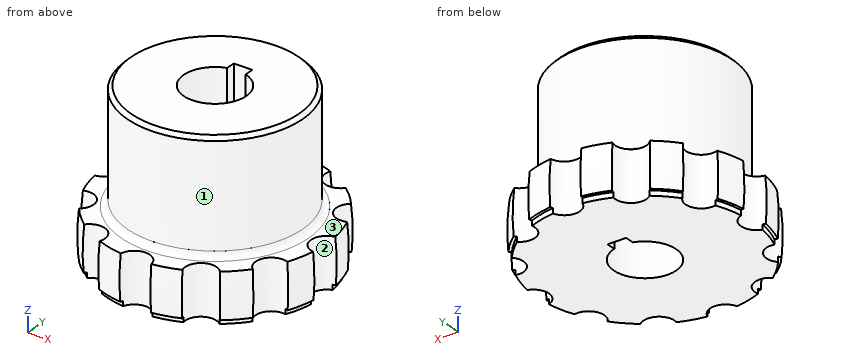
from build123d import *

# Parameters (mm, degrees)
SKETCH_1_R          = 130
EXTRUDE_1_DEPTH     = 40
SKETCH_2_R          = 70
EXTRUDE_2_DEPTH     = 130
SKETCH_4_R          = 12.5
CUT_EXTRUDE_1_DEPTH = 70
FILLET_1_R          = 5
CHAMFER_1_SIZE      = 3
SCALE_1_SCALE       = 0.2
CUT_EXTRUDE_3_DEPTH = 37.215474988


with BuildPart() as part:
    # 草图1 → 凸台-拉伸1 (new body)
    with BuildSketch(Plane.XY):
        Circle(SKETCH_1_R)
    extrude(amount=EXTRUDE_1_DEPTH)

    # 草图2 → 凸台-拉伸2 (add)
    with BuildSketch(Plane.XY):
        Circle(SKETCH_2_R)
    extrude(amount=EXTRUDE_2_DEPTH)

    # 草图3 → 切除-旋转1 (revolve, cut)
    with BuildSketch(Plane(origin=(0, 0, 0), x_dir=(1, 0, 0), z_dir=(0, 1, 0))):
        with BuildLine():
            Line((-87, 0), (-87, -4))
            Line((-87, -4), (-89.287478648, -4))
            ThreePointArc((-89.287478648, -4), (-89.988776291, -22.010076897), (-88.8854382, -40))
            Line((-88.8854382, -40), (-140, -40))
            Line((-140, -40), (-140, 0))
            Line((-140, 0), (-87, 0))
        make_face()
    revolve(axis=Axis((0, 0, -59.373086337), (0, 0, 1)), mode=Mode.SUBTRACT)

    # 草图4 → 切除-拉伸1 (cut)
    with BuildSketch(Plane.XY.offset(40)):
        with Locations((0, 90)):
            Circle(SKETCH_4_R)
        with Locations((45, 77.942286341)):
            Circle(SKETCH_4_R)
        with Locations((77.942286341, 45)):
            Circle(SKETCH_4_R)
        with Locations((90, 0)):
            Circle(SKETCH_4_R)
        with Locations((77.942286341, -45)):
            Circle(SKETCH_4_R)
        with Locations((45, -77.942286341)):
            Circle(SKETCH_4_R)
        with Locations((0, -90)):
            Circle(SKETCH_4_R)
        with Locations((-45, -77.942286341)):
            Circle(SKETCH_4_R)
        with Locations((-77.942286341, -45)):
            Circle(SKETCH_4_R)
        with Locations((-90, 0)):
            Circle(SKETCH_4_R)
        with Locations((-77.942286341, 45)):
            Circle(SKETCH_4_R)
        with Locations((-45, 77.942286341)):
            Circle(SKETCH_4_R)
    extrude(amount=-CUT_EXTRUDE_1_DEPTH, mode=Mode.SUBTRACT)

    # 圆角1
    fillet_1_edges = [part.edges().sort_by_distance(p)[0] for p in [
        (-70, 0, 40),
    ]]
    fillet(fillet_1_edges, radius=FILLET_1_R)

    # 倒角1
    chamfer_1_edges = [part.edges().sort_by_distance(p)[0] for p in [
        (-70, 0, 130),
    ]]
    chamfer(chamfer_1_edges, length=CHAMFER_1_SIZE)


with BuildPart() as part_1:
    # 缩放比例1: scaled about (0, 0, 59.385771994)
    add(part.part.scale(SCALE_1_SCALE).moved(Location((0, 0, 47.508617595))))

    # 草图8 → 切除-拉伸3 (cut, through all)
    with BuildSketch(Plane.XY.offset(73.508624031)):
        with BuildLine():
            Line((1.5, 4.769696007), (1.5, 6.269696007))
            Line((1.5, 6.269696007), (-1.5, 6.269696007))
            Line((-1.5, 6.269696007), (-1.5, 4.769696007))
            ThreePointArc((-1.5, 4.769696007), (0, -5), (1.5, 4.769696007))
        make_face()
    extrude(amount=-CUT_EXTRUDE_3_DEPTH, mode=Mode.SUBTRACT)


solid = part_1.part
Read the model definition and answer for the solid it produces. Units are mm, in the model's axes. Face numbers are marked on the shaded views. Coordinates: 2 decimals unless noted, no trailing zeros. Loops run counter-clockwise (first coordinate to the right, second up) from the corner with the lowest first, then second, coordinate; pieces in that order, holes last. Notation, with made-up numbers: (10, 65.25) -> (44, 65.25) arc R18 ccw to (44, 74.25) -> close; hole circle Ø6 at (39.25, 20.25). An arc over 180 degrees is marked (long way). Answer in a Markdown table with one row per item.
Item 1: Straight lines are drawn through the part: line 1 along X through (y, z) = (0, 62); line 2 along Y through (x, z) = (0, 61); line 3 along X through (y, z) = (0, 54). For each, find the intervals that lie inside material, in ascending order. Write a range as [from, to].
Returned:
| item | result |
|---|---|
| line 1 | x = [-14, -5], [5, 14] |
| line 2 | y = [-14, -5], [6.27, 14] |
| line 3 | x = [-15.5, -5], [5, 15.5] |
Item 2: For a pull along Y with two mould halves and no side action, classify the marked faces 1, 2 and 3 as released by +Y, released by -Y, zero draft, split by the parting line, or undercut.
Returned:
| item | result |
|---|---|
| face 1 | split by the parting line |
| face 2 | undercut |
| face 3 | zero draft |
Item 3: A cutting plane is placed at A-A on y = 0. Determine the outline of the cut face in (x, z), plus the area to 3 significant figures.
Returned:
| item | result |
|---|---|
| outline | (-15.5, 47.51) -> (-5, 47.51) -> (-5, 73.51) -> (-13.4, 73.51) -> (-14, 72.91) -> (-14, 56.51) arc R1 cw to (-15, 55.51) -> (-15.5, 55.51) -> close; (5, 47.51) -> (15.5, 47.51) -> (15.5, 55.51) -> (15, 55.51) arc R1 cw to (14, 56.51) -> (14, 72.91) -> (13.4, 73.51) -> (5, 73.51) -> close |
| area | 492 mm^2 |
Item 4: A cutting plane is placed at B-B on x = 0. Determine the outline of the cut face in (y, z), plus the area to 3 significant figures.
Returned:
| item | result |
|---|---|
| outline | (-15.5, 47.51) -> (-5, 47.51) -> (-5, 73.51) -> (-13.4, 73.51) -> (-14, 72.91) -> (-14, 56.51) arc R1 cw to (-15, 55.51) -> (-15.5, 55.51) -> close; (6.27, 47.51) -> (15.5, 47.51) -> (15.5, 55.51) -> (15, 55.51) arc R1 cw to (14, 56.51) -> (14, 72.91) -> (13.4, 73.51) -> (6.27, 73.51) -> close |
| area | 459 mm^2 |
Item 5: Each of these flat-tipped pins is pushed along its axis until it touches: P1, Ø10, axis at x = 2, z = 67.5, coming from the +Y side; P2, Ø1.2, axis at y = 5.5, z = 67, coming from the -X side; P3, Ø1, axis at x = -13, y = -12.5, coming from the -Z side; P4, Ø8, axis at x = 0, y = 0, coming from the -Z side. Where does it stop, or does it pass through?
Returned:
| item | result |
|---|---|
| P1 | stops at y = 14 |
| P2 | stops at x = -13.11 |
| P3 | stops at z = 48.31 |
| P4 | passes through |
Item 6: A cutting plane is placed at C-C on z = 69.25. Determine the outline of the cut face in (x, y), plus the area to 3 significant figures.
Returned:
| item | result |
|---|---|
| outline | circle Ø28 at (0, 0); hole (-1.5, 4.77) arc R5 ccw (long way) to (1.5, 4.77) -> (1.5, 6.27) -> (-1.5, 6.27) -> close |
| area | 533 mm^2 |
